Geometry check sheet. Reference: the model listing, model coordinates, mm. A direction names the side the tool comes from. Round coordinates to 2 decimals unless told otherwise and drop trailing zeros. Loops run counter-clockwise (first coordinate to the right, second up) from the corner with the lowest first, then second, coordinate; pieces in that order, holes last.
```python
from build123d import *

# Parameters (mm, degrees)
SKETCH_1_W               = 18
SKETCH_1_H               = 18
SKETCH_1_W_2             = 12.4
SKETCH_1_H_2             = 12.4
EXTRUDE_1_DEPTH          = 15
SKETCH_2_W               = 18
SKETCH_2_H               = 18
EXTRUDE_1_2_DEPTH        = 2.5
FILLET_1_R               = 3
SKETCH_3_W               = 18
SKETCH_3_H               = 7
EXTRUDE_2_DEPTH          = 36.83
FILLET_2_R               = 7.5
FILLET_3_R               = 3
CUT_EXTRUDE_1_DEPTH      = 37
CUT_EXTRUDE_1_DEPTH_BACK = 37
SKETCH_6_R               = 1.6
FILLET_4_R               = 3


# Some blends are built 0.0001 mm under size
with BuildPart() as part:
    # 草图1 → Extrude 1 (new body)
    with BuildSketch(Plane(origin=(0, 0, 0), x_dir=(1, 0, 0), z_dir=(0, 1, 0))):
        Rectangle(SKETCH_1_W, SKETCH_1_H)
        Rectangle(SKETCH_1_W_2, SKETCH_1_H_2, mode=Mode.SUBTRACT)
    extrude(amount=EXTRUDE_1_DEPTH)

    # 草图2 → Extrude 1 2 (add)
    with BuildSketch(Plane(origin=(0, 15, 0), x_dir=(1, 0, 0), z_dir=(0, 1, 0))):
        Rectangle(SKETCH_2_W, SKETCH_2_H)
    extrude(amount=EXTRUDE_1_2_DEPTH)

    # 圆角1
    fillet_1_edges = [part.edges().sort_by_distance(p)[0] for p in [
        (-9, 17.5, 0),
        (0, 17.5, 9),
        (9, 17.5, 0),
        (0, 17.5, -9),
    ]]
    fillet(fillet_1_edges, radius=FILLET_1_R)

    # 草图3 → 凸台-拉伸2 (add)
    with BuildSketch(Plane.XY.offset(9)):
        with Locations((0, 3.5)):
            Rectangle(SKETCH_3_W, SKETCH_3_H)
    extrude(amount=EXTRUDE_2_DEPTH)

    # 圆角2
    fillet_2_edges = [part.edges().sort_by_distance(p)[0] for p in [
        (0, 7, 9),
    ]]
    fillet(fillet_2_edges, radius=FILLET_2_R - 0.0001)  # a hair under: the kernel refuses the full size

    # 圆角3
    # the kernel refuses this fillet: 3 mm, written as the material it takes off along each edge
    with BuildSketch(Plane(origin=(6, 14.5, -6), x_dir=(0, 0, -1), z_dir=(1, 0, 0))) as fillet_3_piece_1_section:
        Polygon((0, 0), (FILLET_3_R, 0), (FILLET_3_R, FILLET_3_R), (0, FILLET_3_R), align=None)
    fillet_3_piece_1 = extrude(amount=FILLET_3_R, mode=Mode.PRIVATE)
    fillet_3_piece_1 = fillet_3_piece_1 - Plane(origin=(6, 14.5, -6), x_dir=(0, -0.7071067811865475, 0.7071067811865475), z_dir=(1, 0, 0)) * Sphere(FILLET_3_R, mode=Mode.PRIVATE)
    add(fillet_3_piece_1, mode=Mode.SUBTRACT)
    with BuildSketch(Plane(origin=(-6, 14.5, -6), x_dir=(0, 0, -1), z_dir=(-1, 0, 0))) as fillet_3_piece_2_section:
        Polygon((0, 0), (FILLET_3_R, 0), (FILLET_3_R, -FILLET_3_R), (0, -FILLET_3_R), align=None)
    fillet_3_piece_2 = extrude(amount=FILLET_3_R, mode=Mode.PRIVATE)
    fillet_3_piece_2 = fillet_3_piece_2 - Plane(origin=(-6, 14.5, -6), x_dir=(0, -0.7071067811865475, 0.7071067811865475), z_dir=(-1, 0, 0)) * Sphere(FILLET_3_R, mode=Mode.PRIVATE)
    add(fillet_3_piece_2, mode=Mode.SUBTRACT)
    with BuildSketch(Plane(origin=(-9, 14.5, -9), x_dir=(0, 0, 1), z_dir=(0, -1, 0)), Plane(origin=(9, -7.5, -9), x_dir=(0, 0, 1), z_dir=(0, 1, 0))) as fillet_3_piece_3:
        with BuildLine():
            CenterArc((FILLET_3_R, -FILLET_3_R), FILLET_3_R, 90, 90)
            Line((0, -FILLET_3_R), (0, 0))
            Line((0, 0), (FILLET_3_R, 0))
        make_face()
    extrude(amount=22, mode=Mode.SUBTRACT)

    # 草图6 → 切除-拉伸1 (cut, two sides: drawn at the far end of the back side and taken through both)
    with BuildSketch(Plane(origin=(-6.2, 0, 0), x_dir=(0, 0, -1), z_dir=(1, 0, 0)).offset(-CUT_EXTRUDE_1_DEPTH_BACK)):
        with Locations((0, 7.5)):
            Circle(SKETCH_6_R)
    extrude(amount=CUT_EXTRUDE_1_DEPTH + CUT_EXTRUDE_1_DEPTH_BACK, mode=Mode.SUBTRACT)

    # 镜向1: part across plane


with BuildPart() as part_1:
    add(part.part)
    add(part.part.mirror(Plane(origin=(0, 0, 45.83), x_dir=(1, 0, 0), z_dir=(0, 0, -1))))

    # 圆角4
    # the kernel refuses this fillet: 3 mm, written as the material it takes off along each edge
    with BuildSketch(Plane(origin=(6, 14.5, 85.66), x_dir=(0, 0, -1), z_dir=(1, 0, 0))) as fillet_4_piece_1_section:
        Polygon((0, 0), (FILLET_4_R, 0), (FILLET_4_R, FILLET_4_R), (0, FILLET_4_R), align=None)
    fillet_4_piece_1 = extrude(amount=FILLET_4_R, mode=Mode.PRIVATE)
    fillet_4_piece_1 = fillet_4_piece_1 - Plane(origin=(6, 14.5, 85.66), x_dir=(0, -0.7071067811865475, 0.7071067811865475), z_dir=(1, 0, 0)) * Sphere(FILLET_4_R, mode=Mode.PRIVATE)
    add(fillet_4_piece_1, mode=Mode.SUBTRACT)
    with BuildSketch(Plane(origin=(6, 14.5, 6), x_dir=(1, 0, 0), z_dir=(0, 0, 1))) as fillet_4_piece_2_section:
        Polygon((0, 0), (FILLET_4_R, 0), (FILLET_4_R, FILLET_4_R), (0, FILLET_4_R), align=None)
    fillet_4_piece_2 = extrude(amount=FILLET_4_R, mode=Mode.PRIVATE)
    fillet_4_piece_2 = fillet_4_piece_2 - Plane(origin=(6, 14.5, 6), x_dir=(-0.7071067811865475, -0.7071067811865475, 0), z_dir=(0, 0, 1)) * Sphere(FILLET_4_R, mode=Mode.PRIVATE)
    add(fillet_4_piece_2, mode=Mode.SUBTRACT)
    with BuildSketch(Plane(origin=(-6, 14.5, 85.66), x_dir=(-1, 0, 0), z_dir=(0, 0, -1))) as fillet_4_piece_3_section:
        Polygon((0, 0), (FILLET_4_R, 0), (FILLET_4_R, FILLET_4_R), (0, FILLET_4_R), align=None)
    fillet_4_piece_3 = extrude(amount=FILLET_4_R, mode=Mode.PRIVATE)
    fillet_4_piece_3 = fillet_4_piece_3 - Plane(origin=(-6, 14.5, 85.66), x_dir=(0.7071067811865475, -0.7071067811865475, 0), z_dir=(0, 0, -1)) * Sphere(FILLET_4_R, mode=Mode.PRIVATE)
    add(fillet_4_piece_3, mode=Mode.SUBTRACT)
    with BuildSketch(Plane(origin=(-6, 14.5, 6), x_dir=(-1, 0, 0), z_dir=(0, 0, 1))) as fillet_4_piece_4_section:
        Polygon((0, 0), (FILLET_4_R, 0), (FILLET_4_R, -FILLET_4_R), (0, -FILLET_4_R), align=None)
    fillet_4_piece_4 = extrude(amount=FILLET_4_R, mode=Mode.PRIVATE)
    fillet_4_piece_4 = fillet_4_piece_4 - Plane(origin=(-6, 14.5, 6), x_dir=(0.7071067811865475, -0.7071067811865475, 0), z_dir=(0, 0, 1)) * Sphere(FILLET_4_R, mode=Mode.PRIVATE)
    add(fillet_4_piece_4, mode=Mode.SUBTRACT)
    with BuildSketch(Plane(origin=(9, 14.4999, 75.1601), x_dir=(0, 0, 1), z_dir=(0, 1, 0))) as fillet_4_piece_5:
        with BuildLine():
            CenterArc((7.4999 + FILLET_4_R, -FILLET_4_R), FILLET_4_R, 90, 90)
            Line((7.4999, -FILLET_4_R), (7.4999, 0))
            Line((7.4999, 0), (7.4999 + FILLET_4_R, 0))
        make_face()
    revolve(axis=Axis((9, 14.4999, 75.1601), (1, 0, 0)), revolution_arc=90, mode=Mode.SUBTRACT)
    with BuildSketch(Plane(origin=(-9, 14.4999, 75.1601), x_dir=(0, 0, 1), z_dir=(0, 1, 0))) as fillet_4_piece_6:
        with BuildLine():
            CenterArc((7.4999 + FILLET_4_R, FILLET_4_R), FILLET_4_R, 180, 90)
            Line((7.4999 + FILLET_4_R, 0), (7.4999, 0))
            Line((7.4999, 0), (7.4999, FILLET_4_R))
        make_face()
    revolve(axis=Axis((-9, 14.4999, 75.1601), (1, 0, 0)), revolution_arc=90, mode=Mode.SUBTRACT)
    with BuildSketch(Plane(origin=(9, 14.4999, 16.4999), x_dir=(0, 0, -1), z_dir=(0, 1, 0))) as fillet_4_piece_7:
        with BuildLine():
            CenterArc((7.4999 + FILLET_4_R, FILLET_4_R), FILLET_4_R, 180, 90)
            Line((7.4999, FILLET_4_R), (7.4999, 0))
            Line((7.4999, 0), (7.4999 + FILLET_4_R, 0))
        make_face()
    revolve(axis=Axis((9, 14.4999, 16.4999), (-1, 0, 0)), revolution_arc=90, mode=Mode.SUBTRACT)
    with BuildSketch(Plane(origin=(-9, 14.4999, 16.4999), x_dir=(0, 0, -1), z_dir=(0, 1, 0))) as fillet_4_piece_8:
        with BuildLine():
            CenterArc((7.4999 + FILLET_4_R, -FILLET_4_R), FILLET_4_R, 90, 90)
            Line((7.4999 + FILLET_4_R, 0), (7.4999, 0))
            Line((7.4999, 0), (7.4999, -FILLET_4_R))
        make_face()
    revolve(axis=Axis((-9, 14.4999, 16.4999), (-1, 0, 0)), revolution_arc=90, mode=Mode.SUBTRACT)
    with BuildSketch(Plane(origin=(9, 0, 97.66), x_dir=(0, 1, 0), z_dir=(0, 0, -1))) as fillet_4_piece_9:
        with BuildLine():
            CenterArc((FILLET_4_R, -FILLET_4_R), FILLET_4_R, 90, 90)
            Line((0, -FILLET_4_R), (0, 0))
            Line((0, 0), (FILLET_4_R, 0))
        make_face()
    extrude(amount=103.66, mode=Mode.SUBTRACT)
    with BuildSketch(Plane(origin=(-9, 0, -6), x_dir=(1, 0, 0), z_dir=(0, 0, 1))) as fillet_4_piece_10:
        with BuildLine():
            CenterArc((FILLET_4_R, FILLET_4_R), FILLET_4_R, 180, 90)
            Line((0, FILLET_4_R), (0, 0))
            Line((0, 0), (FILLET_4_R, 0))
        make_face()
    extrude(amount=103.66, mode=Mode.SUBTRACT)
    with BuildSketch(Plane(origin=(9, 7, 16.4999), x_dir=(0, -1, 0), z_dir=(0, 0, 1))) as fillet_4_piece_11:
        with BuildLine():
            CenterArc((FILLET_4_R, -FILLET_4_R), FILLET_4_R, 90, 90)
            Line((0, -FILLET_4_R), (0, 0))
            Line((0, 0), (FILLET_4_R, 0))
        make_face()
    extrude(amount=58.6602, mode=Mode.SUBTRACT)
    with BuildSketch(Plane(origin=(-9, 7, 75.1601), x_dir=(1, 0, 0), z_dir=(0, 0, -1))) as fillet_4_piece_12:
        with BuildLine():
            CenterArc((FILLET_4_R, FILLET_4_R), FILLET_4_R, 180, 90)
            Line((0, FILLET_4_R), (0, 0))
            Line((0, 0), (FILLET_4_R, 0))
        make_face()
    extrude(amount=58.6602, mode=Mode.SUBTRACT)
    with BuildSketch(Plane(origin=(-6, 0, -6), x_dir=(0, 0, -1), z_dir=(1, 0, 0))) as fillet_4_piece_13:
        with BuildLine():
            CenterArc((3 - FILLET_4_R, FILLET_4_R), FILLET_4_R, 270, 90)
            Line((3 - FILLET_4_R, 0), (3, 0))
            Line((3, 0), (3, FILLET_4_R))
        make_face()
    revolve(axis=Axis((-6, 0, -6), (0, 1, 0)), revolution_arc=90, mode=Mode.SUBTRACT)
    with BuildSketch(Plane(origin=(-6, 0, 97.66), x_dir=(0, 0, 1), z_dir=(1, 0, 0))) as fillet_4_piece_14:
        with BuildLine():
            CenterArc((3 - FILLET_4_R, -FILLET_4_R), FILLET_4_R, 0, 90)
            Line((3, -FILLET_4_R), (3, 0))
            Line((3, 0), (3 - FILLET_4_R, 0))
        make_face()
    revolve(axis=Axis((-6, 0, 97.66), (0, -1, 0)), revolution_arc=90, mode=Mode.SUBTRACT)
    with BuildSketch(Plane(origin=(-6, 0, 100.66), x_dir=(0, 0, -1), z_dir=(1, 0, 0)), Plane(origin=(-6, 0, -9), x_dir=(0, 1, 0), z_dir=(1, 0, 0))) as fillet_4_piece_15:
        with BuildLine():
            CenterArc((FILLET_4_R, FILLET_4_R), FILLET_4_R, 180, 90)
            Line((0, FILLET_4_R), (0, 0))
            Line((0, 0), (FILLET_4_R, 0))
        make_face()
    extrude(amount=12, mode=Mode.SUBTRACT)
    with BuildSketch(Plane(origin=(6, 0, 97.66), x_dir=(0, 0, 1), z_dir=(-1, 0, 0))) as fillet_4_piece_16:
        with BuildLine():
            CenterArc((3 - FILLET_4_R, FILLET_4_R), FILLET_4_R, 270, 90)
            Line((3, FILLET_4_R), (3, 0))
            Line((3, 0), (3 - FILLET_4_R, 0))
        make_face()
    revolve(axis=Axis((6, 0, 97.66), (0, 1, 0)), revolution_arc=90, mode=Mode.SUBTRACT)
    with BuildSketch(Plane(origin=(6, 0, -6), x_dir=(0, 0, -1), z_dir=(-1, 0, 0))) as fillet_4_piece_17:
        with BuildLine():
            CenterArc((3 - FILLET_4_R, -FILLET_4_R), FILLET_4_R, 0, 90)
            Line((3 - FILLET_4_R, 0), (3, 0))
            Line((3, 0), (3, -FILLET_4_R))
        make_face()
    revolve(axis=Axis((6, 0, -6), (0, -1, 0)), revolution_arc=90, mode=Mode.SUBTRACT)
    with BuildSketch(Plane(origin=(-9, 14.5, 9), x_dir=(1, 0, 0), z_dir=(0, -1, 0)), Plane(origin=(9, 14.4999, 9), x_dir=(-1, 0, 0), z_dir=(0, 1, 0)), Plane(origin=(9, 14.4999, 82.66), x_dir=(0, 0, 1), z_dir=(0, 1, 0))) as fillet_4_piece_18:
        with BuildLine():
            CenterArc((FILLET_4_R, -FILLET_4_R), FILLET_4_R, 90, 90)
            Line((0, -FILLET_4_R), (0, 0))
            Line((0, 0), (FILLET_4_R, 0))
        make_face()
    extrude(amount=0.0001, mode=Mode.SUBTRACT)
    with BuildSketch(Plane(origin=(-9, 14.5, 82.66), x_dir=(1, 0, 0), z_dir=(0, -1, 0))) as fillet_4_piece_19:
        with BuildLine():
            CenterArc((FILLET_4_R, FILLET_4_R), FILLET_4_R, 180, 90)
            Line((0, FILLET_4_R), (0, 0))
            Line((0, 0), (FILLET_4_R, 0))
        make_face()
    extrude(amount=0.0001, mode=Mode.SUBTRACT)


solid = part_1.part
```
1) Access from +Z, -Z, +X, -X, +Y, -Y to the whole of each face (thin tool, end or side, straight path). Record for faces 5 (the face through (8.14, 16.6, 91.74)), 6 (the face through (8.14, 6.1, 45.42)), 7 (the face through (0, 7, 46)), 8 (the face through (6.2, 5.7, 0.1)).
Report:
face 5: +Z, -Z, +X, +Y
face 6: +X, +Y
face 7: +X, -X, +Y
face 8: -Y
2) Scan lines: line 1 along Z through (x, y) = (6, 5.5); line 2 along X through (y, z) = (12, 87.5); line 3 along Z through (x, y) = (-8.1, 7.5). Record each from-to range of solid material in increasing order.
Report:
line 1: z = -9 to -6.2, 6.2 to 85.46, 97.86 to 100.66
line 2: x = -9 to -6.2, 6.2 to 9
line 3: z = -8.14 to -1.6, 1.6 to 11.93, 79.73 to 90.06, 93.26 to 99.8
3) Sectioned sample at C-C, the plane y = 16. Record the cut outline in (x, z), then the cut area to 3 significant figures.
Report:
outline: (-8.6, -6) arc R2.6 ccw to (-6, -8.6) - (6, -8.6) arc R2.6 ccw to (8.6, -6) - (8.6, 6) arc R2.6 ccw to (6, 8.6) - (-6, 8.6) arc R2.6 ccw to (-8.6, 6) - close; (-8.6, 85.66) arc R2.6 ccw to (-6, 83.06) - (6, 83.06) arc R2.6 ccw to (8.6, 85.66) - (8.6, 97.66) arc R2.6 ccw to (6, 100.26) - (-6, 100.26) arc R2.6 ccw to (-8.6, 97.66) - close
area: 580 mm2
4) Mould release check, pull along Z, two halves, no side actions. Record for faces 1 (the face through (0, 9, 100.66)), 2 (the face through (-8.14, 0.9, 45.1)), 3 (the face through (6.2, 5.7, 91.6)), 4 (the face through (-7.62, 5.94, 0.35)): +Z half, -Z half, draft (parallel to the pull), parting line (faces both ways), or undercut.
Report:
face 1: +Z half
face 2: draft
face 3: undercut
face 4: undercut
5) Sectioned sample at D-D, the plane z = 33. Record the cut outline in (x, y), then the cut area to 3 significant figures.
Report:
outline: (-9, 3) arc R3 ccw to (-6, 0) - (6, 0) arc R3 ccw to (9, 3) - (9, 4) arc R3 ccw to (6, 7) - (-6, 7) arc R3 ccw to (-9, 4) - close
area: 118 mm2
6) Sectioned sample at A-A, the plane z = 0. Record the cut outline in (x, y).
Report:
outline: (-9, 3) arc R3 ccw to (-6.2, 0.01) - (-6.2, 5.9) - (-9, 5.9) - close; (-9, 9.1) - (-6.2, 9.1) - (-6.2, 15) - (6.2, 15) - (6.2, 9.1) - (9, 9.1) - (9, 14.5) arc R3 ccw to (6, 17.5) - (-6, 17.5) arc R3 ccw to (-9, 14.5) - close; (6.2, 0.01) arc R3 ccw to (9, 3) - (9, 5.9) - (6.2, 5.9) - close
7) Gauge pin test, flat ends, axial feed: pin 1 (3 mm diameter, centred on y = 7.5, z = 91.66, fed in from -X); pin 2 (2 mm diameter, centred on y = 6.5, z = 66.5, fed in from -X); pin 3 (10 mm diameter, centred on x = 4, z = 21.5, fed in from +Y). Record the tip position at first contact, or that the pin passes through.
Report:
pin 1: passes through
pin 2: stops at x = -8.6
pin 3: stops at y = 7
8) Sectioned sample at B-B, the plane x = 7.5. State how many separate pieces and enclosed holes the cut face has, then the cut area to 3 significant figures.
Report:
separate pieces: 1
enclosed holes: 2
area: 1,040 mm2
